Input: part model. Units: mm. Frame: model coordinates. Coordinates: 2 decimals unless noted, no trailing zeros. Order: outer loops, then holes, each group sorted by start corner. A loop starts at its lowest first (then second) coordinate and runs counter-clockwise, first axis right, second up. Notation, with made-up numbers: (50, -15) - (105, -15) arc R31 cw to (105, 18) - close; hole circle Ø9 at (-37, 61). An arc over 180 degrees is marked (long way). Answer as CSV lines item,"result". Start each with the question number.
Item 1: Material intervals for line 1 along Z through (x, y) = (-47.4, 182); line 2 along Y through (x, z) = (-47.65, 100); line 3 along Z through (x, y) = (-48.9, 134), sorted ascending.
Item 2: Section A-A (y = 200.5). Output: boundary loops of the cut face in (x, z), and give its area (3 significant figures).
Item 3: Section B-B (x = -47). Output: boundary loops of the cut face in (y, z).
Item 4: Section D-D (y = 188). Output: boundary loops of the cut face in (x, z).
Item 5: First-contact query: pin 1 (1 mm diameter, centred on x = -48, z = 121, fed in from -Y); pin 2 (1 mm diameter, centred on x = -47, y = 168, fed in from +Z). Flat tips, straight axial feed; report the tip coordinate or a pass-through.
Item 6: Section C-C (z = 118). Output: boundary loops of the cut face in (x, y), and give its area (3 significant figures).
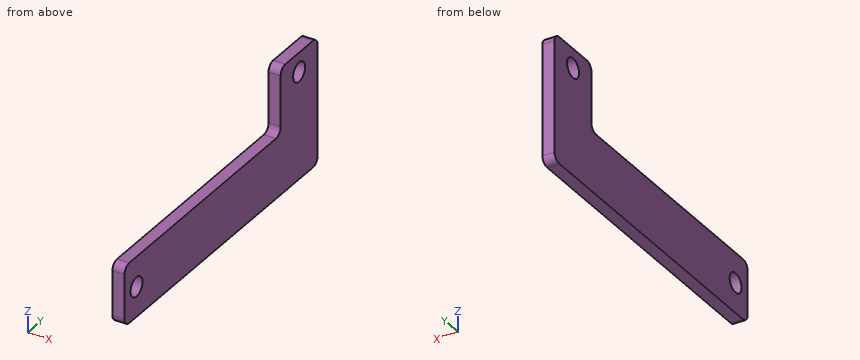
from build123d import *

# Parameters (mm, degrees)
BASE_FLANGE1_DEPTH = 3.175
SKETCH9_R          = 2.54
CUT_EXTRUDE2_DEPTH = 246.387748173
FILLET1_R          = 2


# Sheet-metal steps are written as plain solids
with BuildPart() as part:
    # Sketch2 → Base-Flange1 (new body)
    with BuildSketch(Plane(origin=(-49.425032983, 0, 0), x_dir=(0, 0, -1), z_dir=(1, 0, 0))):
        Polygon((-94.005448243, 127.917372069), (-109.749301699, 127.917372069), (-109.749301699, 194.197401704), (-127.122990112, 194.197401704), (-127.122990112, 209.868558182), (-109.749301699, 209.868558182), (-94.005448243, 209.868558182), align=None)
    extrude(amount=BASE_FLANGE1_DEPTH)

    # Sketch9 → Cut-Extrude2 (cut, through all)
    with BuildSketch(Plane.ZY.offset(49.425032983)):
        with Locations(Location((122.042990112, 202.032979943, 0), (0, 0, 270))):
            Circle(SKETCH9_R)
        with Locations(Location((101.877374971, 132.997372069, 0), (0, 0, 270))):
            Circle(SKETCH9_R)
    extrude(amount=-CUT_EXTRUDE2_DEPTH, mode=Mode.SUBTRACT)

    # Fillet1
    fillet1_edges = [part.edges().sort_by_distance(p)[0] for p in [
        (-47.837532983, 127.917372069, 94.005448243),
        (-47.837532983, 127.917372069, 109.749301699),
        (-47.837532983, 194.197401704, 109.749301699),
        (-47.837532983, 194.197401704, 127.122990112),
        (-47.837532983, 209.868558182, 127.122990112),
        (-47.837532983, 209.868558182, 94.005448243),
    ]]
    fillet(fillet1_edges, radius=FILLET1_R)


solid = part.part
Determined:
1,line 1,"z = 94.01 to 109.75"
1,line 2,"y = 127.92 to 131.29, 134.71 to 209.87"
1,line 3,"z = 94.01 to 99.54, 104.21 to 109.75"
2,outline,"(-49.43, 94.01) - (-46.25, 94.01) - (-46.25, 120.02) - (-49.43, 120.02) - close; (-49.43, 124.07) - (-46.25, 124.07) - (-46.25, 127.12) - (-49.43, 127.12) - close"
2,area,"92.3 mm^2"
3,outline,"(127.92, 96.01) arc R2 ccw to (129.92, 94.01) - (207.87, 94.01) arc R2 ccw to (209.87, 96.01) - (209.87, 125.12) arc R2 ccw to (207.87, 127.12) - (196.2, 127.12) arc R2 ccw to (194.2, 125.12) - (194.2, 111.75) arc R2 cw to (192.2, 109.75) - (129.92, 109.75) arc R2 ccw to (127.92, 107.75) - close; hole circle Ø5.08 at (133, 101.88); hole circle Ø5.08 at (202.03, 122.04)"
4,outline,"(-49.43, 94.01) - (-46.25, 94.01) - (-46.25, 109.75) - (-49.43, 109.75) - close"
5,pin 1,"stops at y = 194.2"
5,pin 2,"stops at z = 109.75"
6,outline,"(-49.43, 194.2) - (-46.25, 194.2) - (-46.25, 209.87) - (-49.43, 209.87) - close"
6,area,"49.8 mm^2"
